Geometry: final body of the model. Coordinates: model frame, mm. Give positions to 0.01 mm unless a question says otherwise; leave off trailing zeros. Write each loop counter-clockwise with the first axis right and the second up, starting at its lowest first coordinate (ties: lowest second). Pieces come first, ordered by that corner, then holes.
Q1. Cut plane A-A on z = 12.5. Return the cut outline in (x, y), plus the area to 3 significant figures.
Q2. Pin query (flat end, axial travel): pin 1 (4 mm diameter, centred on x = -417, z = 6, fed in from -Y); pin 2 (10 mm diameter, centred on y = 150.5, z = 7, fed in from +X); pin 3 (5 mm diameter, centred on y = 18.5, z = 7.5, fed in from -X). Return the tip coordinate at first contact, or that it passes through.
Q3. Line query: L1, parallel to Y at x = -870, z = 3.25; L2, parallel to Y at x = -287, z = 6.75; L3, parallel to X at y = 53, z = 2. Output: solid intervals per line, ascending.
```python
from build123d import *

# Parameters (mm, degrees)
F1_DEPTH = 19.05
F2_SIZE  = 19.04999


# Not quite as in the source:
# - a fillet or chamfer is up to 0.001 mm smaller than in the source, because OpenCascade refuses the exact size


with BuildPart() as f1:
    # F0 (on Top) → F1 (new body)
    with BuildSketch(Plane.XY):
        Polygon((-1155.7, -190.5), (1155.7, -190.5), (1155.7, 190.5), (946.15, 190.5), (946.15, 171.45), (-946.15, 171.45), (-946.15, 190.5), (-1155.7, 190.5), align=None)
    extrude(amount=F1_DEPTH)

    # F2 (size 19.05 in the source; OpenCascade refuses exactly that, so slightly less here)
    f2_edges = [f1.edges().sort_by_distance(p)[0] for p in [
        (-1155.7, 0, 0),
        (0, -190.5, 0),
        (1155.7, 0, 0),
    ]]
    chamfer(f2_edges, length=F2_SIZE)


solid = f1.part
```
Data:
1. outline: (-1149.15, -183.95) - (1149.15, -183.95) - (1149.15, 190.5) - (946.15, 190.5) - (946.15, 171.45) - (-946.15, 171.45) - (-946.15, 190.5) - (-1149.15, 190.5) - close
1. area: 825,000 mm2
2. pin 1: stops at y = -179.45
2. pin 2: stops at x = 1148.65
2. pin 3: stops at x = -1146.65
3. L1: y = -174.7 to 171.45
3. L2: y = -178.2 to 171.45
3. L3: x = -1138.65 to 1138.65
